Can you work these out from the model? Positions are in its coordinate system, mm. Face numbers are marked on the shaded views. A direction names the side the tool comes from. Give positions to 0.01 mm unless a question says otherwise; leave off trailing zeros. Order: outer loops, then holes, each group sorted by start corner. A loop starts at its lowest first (then second) coordinate and runs counter-clockwise, first axis right, second up. Notation, with made-up numbers: (18.25, 54) -> (44.25, 54) arc R26 ccw to (44.25, 69) -> close; hole circle Ø10 at (32.5, 41). An arc over 180 degrees is marked (long way). Answer as CSV lines item,"result".
```python
from build123d import *

# Parameters (mm, degrees)
SKETCH1_R               = 1.5
BOSS_EXTRUDE1_DEPTH     = 23
BOSS_EXTRUDE2_START     = 8
SKETCH2_R               = 2.5
BOSS_EXTRUDE2_DEPTH     = 5
BOSS_EXTRUDE3_DEPTH     = 2
BOSS_EXTRUDE4_START     = 4
SKETCH5_R               = 2.5
BOSS_EXTRUDE4_DEPTH     = 1
BOSS_EXTRUDE4_TAPER     = 45
CUT_EXTRUDE1_DEPTH      = 24.613202522
CUT_EXTRUDE1_DEPTH_BACK = 24.613202522
SKETCH6_R               = 1


with BuildPart() as part:
    # Sketch1 → Boss-Extrude1 (new body)
    with BuildSketch(Plane(origin=(0, 0, 0), x_dir=(1, 0, 0), z_dir=(0, 1, 0))):
        with Locations(Location((0, 0, 0), (0, 0, 270))):
            Circle(SKETCH1_R)
    extrude(amount=BOSS_EXTRUDE1_DEPTH)

    # Sketch2 → Boss-Extrude2 (add)
    with BuildSketch(Plane(origin=(0, 0, 0), x_dir=(1, 0, 0), z_dir=(0, 1, 0)).offset(BOSS_EXTRUDE2_START)):
        with Locations(Location((0, 0, 0), (0, 0, 270))):
            Circle(SKETCH2_R)
    extrude(amount=BOSS_EXTRUDE2_DEPTH)

    # Sketch3 → Boss-Extrude3 (add)
    with BuildSketch(Plane(origin=(0, 13, 0), x_dir=(1, 0, 0), z_dir=(0, 1, 0))):
        Polygon((-2.020725942, 3.5), (-4.041451884, 0), (-2.020725942, -3.5), (2.020725942, -3.5), (4.041451884, 0), (2.020725942, 3.5), align=None)
    extrude(amount=BOSS_EXTRUDE3_DEPTH)

    # Sketch5 → Boss-Extrude4 (add)
    with BuildSketch(Plane(origin=(0, 15, 0), x_dir=(1, 0, 0), z_dir=(0, 1, 0)).offset(BOSS_EXTRUDE4_START)):
        with Locations(Location((0, 0, 0), (0, 0, 270))):
            Circle(SKETCH5_R)
    extrude(amount=BOSS_EXTRUDE4_DEPTH, taper=BOSS_EXTRUDE4_TAPER)

    # Sketch6 → Cut-Extrude1 (cut, two sides: drawn at the far end of the back side and taken through both)
    with BuildSketch(Plane.XZ.offset(-CUT_EXTRUDE1_DEPTH_BACK)):
        with Locations(Location((0, 0, 0), (0, 0, 270))):
            Circle(SKETCH6_R)
    extrude(amount=CUT_EXTRUDE1_DEPTH + CUT_EXTRUDE1_DEPTH_BACK, mode=Mode.SUBTRACT)


solid = part.part
```
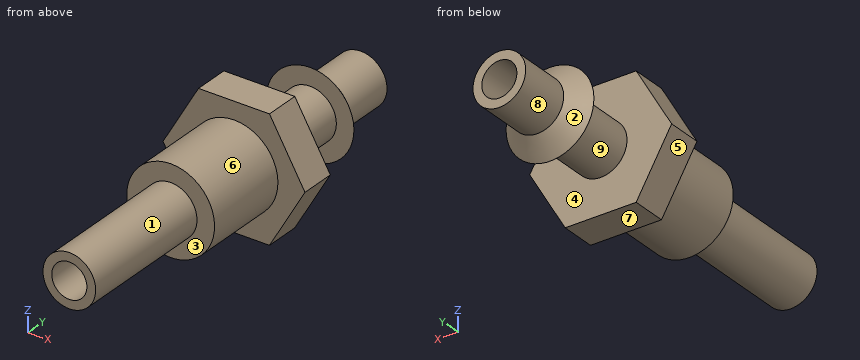
Item 1: For the marked faces 5, 6, 7, 8 and 9, which set-ups out of +Z, -Z, +X, -X, +Y, -Y let a thin tool reach every point of the face, with its end or its side?
Numbers:
face 5,"-Z, -X, +Y, -Y"
face 6,"-Y"
face 7,"-Z, +X, -X, +Y, -Y"
face 8,"+Y"
face 9,"none"
Item 2: Imagine slicing it at B-B, the plane z = 3. Please give me the cut outline in (x, y).
Numbers:
outline,"(-2.31, 13) -> (2.31, 13) -> (2.31, 15) -> (-2.31, 15) -> close"
Item 3: Imagine slicing it at A-A, the plane y = 14. Please give me the cut outline in (x, z).
Numbers:
outline,"(-4.04, 0) -> (-2.02, -3.5) -> (2.02, -3.5) -> (4.04, 0) -> (2.02, 3.5) -> (-2.02, 3.5) -> close; hole circle Ø2 at (0, 0)"
Item 4: For pin 1 (3.5 mm diameter, centred on x = -0.5, z = 0.5, fed in from +Y); pin 2 (4 mm diameter, centred on y = 19, z = 2, fed in from +X); pin 3 (1 mm diameter, centred on x = 3, y = 14.5, fed in from -Z), each with a flat end and sliding along its axis, tell me the tip position at first contact or that it passes through.
Numbers:
pin 1,"stops at y = 23"
pin 2,"stops at x = 2.5"
pin 3,"stops at z = -2.67"
Item 5: Imagine slicing it at D-D, the plane x = 3. Please give me the cut outline in (y, z), then the cut area to 3 significant figures.
Numbers:
outline,"(13, -1.8) -> (15, -1.8) -> (15, 1.8) -> (13, 1.8) -> close"
area,"7.22 mm²"
Item 6: Imagine slicing it at C-C, the plane y = 5.25. Please give me the cut outline in (x, z), then the cut area to 3 significant figures.
Numbers:
outline,"circle Ø3 at (0, 0); hole circle Ø2 at (0, 0)"
area,"3.93 mm²"
Item 7: We'd pull the mould along Y, two halves only. Please class the marked faces 1, 2, 3 and 4: released by +Y, released by -Y, zero draft, split by the parting line, or undercut.
Numbers:
face 1,"zero draft"
face 2,"released by +Y"
face 3,"released by -Y"
face 4,"undercut"
Item 8: Please list where these lines run through material, in increasing order: line 1 along X through (y, z) = (15.25, 0); line 2 along X through (y, z) = (10, 0); line 3 along Y through (x, z) = (2.25, -3).
Numbers:
line 1,"x = -1.5 to -1, 1 to 1.5"
line 2,"x = -2.5 to -1, 1 to 2.5"
line 3,"y = 13 to 15"
